```python
from build123d import *

# Parameters (mm, degrees)
F0_W            = 8
F0_H            = 17.05
F3_D            = 6
F4_T            = -2
F6_D            = 8
F6_COPIES_COUNT = 5
F7_SIZE         = 1


# Not quite as in the source:
# - a pattern or mirror of a feature is missing from the dataset's text; its kind, count and spacing are read off the source's solid


with BuildPart() as f1:
    # F0 (on Top) → F1 (revolve)
    with BuildSketch(Plane.XY):
        with Locations((4, 8.525)):
            Rectangle(F0_W, F0_H)
    revolve(axis=Axis((4, 0, 0), (1, 0, 0)))

    # F3 (through all)
    with Locations(Plane(origin=(0, 0, 0), x_dir=(0, 1, 0), z_dir=(-1, 0, 0))):
        with Locations((0, 0)):
            Hole(F3_D / 2)

    # F4
    f4_openings = [f1.faces().sort_by_distance(p)[0] for p in [
        (8, -16.567753, 0),
    ]]
    offset(amount=F4_T, openings=f4_openings)

    # F6 (through all)
    with Locations(Plane(origin=(0, 0, 0), x_dir=(0, 1, 0), z_dir=(-1, 0, 0))):
        with Locations((0, -10)):
            f6 = Hole(F6_D / 2)

    # F6_copies: F6 ×5 about axis
    f6_copies_axis = Axis((0, 0, 0), (1, 0, 0))
    for i in range(1, F6_COPIES_COUNT):
        add(f6.rotate(f6_copies_axis, i * 360 / F6_COPIES_COUNT), mode=Mode.SUBTRACT)

    # F7
    f7_edges = [f1.edges().sort_by_distance(p)[0] for p in [
        (8, -5, 0),
    ]]
    chamfer(f7_edges, length=F7_SIZE)


solid = f1.part
```
Verification items for the finished model (mm, model axes). A direction names the side the tool comes from. Give positions to 0.01 mm unless a question says otherwise; leave off trailing zeros. Loops run counter-clockwise (first coordinate to the right, second up) from the corner with the lowest first, then second, coordinate; pieces in that order, holes last.
1. Set-up check for faces 1 (the cylindrical face through (1.014, 4.74, -11.925)), 2 (the cylindrical face through (5.042, -3.263, -14.692)): record each of +Z, -Z, +X, -X, +Y, -Y from which the full face is reachable in a straight line by a thin tool's end or side.
2. Section check D-D, the plane z = 11. Enter the section's corners in (x, y), then the cut area to 3 significant figures.
3. Section check C-C, the plane x = 5.25. Enter the section's corners in (y, z).
4. Section check A-A, the plane y = 0. Enter the section's corners in (x, z), then the cut area to 3 significant figures.
5. Go/stop test with flat-tipped pins: pin 1 Ø7 at (y, z) = (0, 10) entering from +X; pin 2 Ø1.5 at (x, y) = (3.5, -1.5) entering from -Z; pin 3 Ø13 at (y, z) = (5.88, -8.09) entering from -X; pin 4 Ø1.5 at (x, y) = (7, -9) entering from -Z. Record where each tip stops, or that it passes through.
6. Thickness scan on line 1 (Z direction, x = 0.75, y = 7); line 2 (Z direction, x = 4.5, y = 2); line 3 (Y direction, x = 4, z = 4). Record the ranges inside material, lowest first.
7. Mould release check, pull along Y, two halves, no side actions. Record for faces 3 (the cylindrical face through (4.54, 1.08, 4.88)), 4 (the flat face through (0, -4, 0)), 5 (the cylindrical face through (4.056, -2.22, 16.905)): released by +Y, released by -Y, zero draft, split by the parting line, or undercut.
8. Section check B-B, the plane z = -10. Enter the section's corners in (x, y).
Geometry says:
1. face 1: +X, -X
1. face 2: +X
2. outline: (0, -13.03) - (8, -13.03) - (8, -10.27) - (2, -10.27) - (2, -3.87) - (0, -3.87) - close; (0, 3.87) - (2, 3.87) - (2, 10.27) - (8, 10.27) - (8, 13.03) - (0, 13.03) - close
2. area: 69.7 mm2
3. outline: circle Ø34.1 at (0, 0); circle Ø10 at (0, 0); hole circle Ø30.1 at (0, 0); hole circle Ø6 at (0, 0)
4. outline: (0, -17.05) - (8, -17.05) - (8, -15.05) - (2, -15.05) - (2, -5) - (7, -5) - (8, -4) - (8, -3) - (0, -3) - close; (0, 3) - (8, 3) - (8, 4) - (7, 5) - (2, 5) - (2, 6) - (0, 6) - close; (0, 14) - (2, 14) - (2, 15.05) - (8, 15.05) - (8, 17.05) - (0, 17.05) - close
4. area: 87.2 mm2
5. pin 1: passes through
5. pin 2: stops at z = -17.03
5. pin 3: stops at x = 0
5. pin 4: stops at z = -14.92
6. line 1: z = -15.55 to -11.93, -4.25 to -0.02, 6.2 to 15.55
6. line 2: z = -16.93 to -14.92, -4.58 to -2.24, 2.24 to 4.58, 14.92 to 16.93
6. line 3: y = -16.57 to -14.51, -3 to 3, 14.51 to 16.57
7. face 3: undercut
7. face 4: zero draft
7. face 5: split by the parting line
8. outline: (0, -13.81) - (8, -13.81) - (8, -11.25) - (2, -11.25) - (2, -9.39) - (0, -9.39) - close; (0, -2.36) - (2, -2.36) - (2, 2.36) - (0, 2.36) - close; (0, 9.39) - (2, 9.39) - (2, 11.25) - (8, 11.25) - (8, 13.81) - (0, 13.81) - close
